Input: part model. Units: mm. Frame: model coordinates. Give positions to 0.01 mm unless a question says otherwise; leave off trailing zeros. Order: outer loops, then holes, each group sorted by start corner. A loop starts at its lowest first (then second) coordinate and runs counter-clockwise, first axis right, second up. Notation, with made-up numbers: (-29, -36) - (0, -36) arc R31 cw to (0, -9) - close; hole circle Ø9 at (7, 18.5). An arc over 180 degrees is marked (long way). Use a Markdown table: item, result.
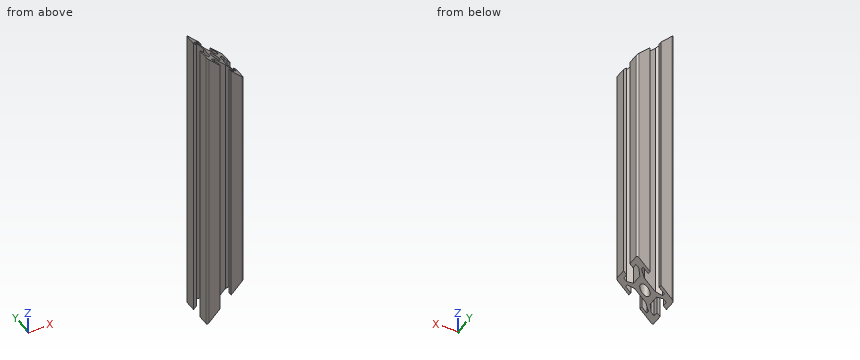
from build123d import *

# Parameters (mm, degrees)
BOSS_EXTRUDE1_DEPTH     = 82.23
CUT_EXTRUDE1_DEPTH      = 166.066930668
CUT_EXTRUDE1_DEPTH_BACK = 166.066930668
SKETCH2_R               = 2.5
FILLET1_R               = 1
SKETCH3_W               = 42.278905999
SKETCH3_H               = 22
CUT_EXTRUDE2_DEPTH      = 128.405385483
SKETCH4_W               = 35
SKETCH4_H               = 22.104489803
CUT_EXTRUDE3_DEPTH      = 128.405385483


with BuildPart() as part:
    # Sketch1 → Boss-Extrude1 (new, symmetric)
    with BuildSketch(Plane.XY):
        Polygon((-10, 10), (-3, 10), (-3, 8.272610059), (-5.783778863, 8.272610059), (-5.783778863, 6.747994248), (-3, 4.550753814), (3, 4.550753814), (5.783778863, 6.747994248), (5.783778863, 8.272610059), (3, 8.272610059), (3, 10), (10, 10), (10, 3), (8.272610059, 3), (8.272610059, 5.783778863), (6.747994248, 5.783778863), (4.55, 3.000595152), (4.55, -2.999404848), (6.747994248, -5.783778863), (8.272610059, -5.783778863), (8.272610059, -3), (10, -3), (10, -10), (3, -10), (3, -8.272610059), (5.783778863, -8.272610059), (5.783778863, -6.747994248), (2.999404848, -4.55), (-3.000595152, -4.55), (-5.783778863, -6.747994248), (-5.783778863, -8.272610059), (-3, -8.272610059), (-3, -10), (-10, -10), (-10, -3), (-8.272610059, -3), (-8.272610059, -5.783778863), (-6.747994248, -5.783778863), (-4.55, -3.000595152), (-4.55, 2.999404848), (-6.747994248, 5.783778863), (-8.272610059, 5.783778863), (-8.272610059, 3), (-10, 3), align=None)
    extrude(amount=BOSS_EXTRUDE1_DEPTH, both=True)

    # Sketch2 → Cut-Extrude1 (cut, two sides: drawn at the far end of the back side and taken through both)
    with BuildSketch(Plane.XY.offset(82.23).offset(-CUT_EXTRUDE1_DEPTH_BACK)):
        Circle(SKETCH2_R)
    extrude(amount=CUT_EXTRUDE1_DEPTH + CUT_EXTRUDE1_DEPTH_BACK, mode=Mode.SUBTRACT)

    # Fillet1
    fillet1_edges = [part.edges().sort_by_distance(p)[0] for p in [
        (-10, 10, 0),
        (10, 10, 0),
        (10, -10, 0),
        (-10, -10, 0),
    ]]
    fillet(fillet1_edges, radius=FILLET1_R)

    # Sketch3 → Cut-Extrude2 (cut, through all)
    with BuildSketch(Plane(origin=(36.115, 0, -36.115), x_dir=(0.7071067811865477, 0, 0.7071067811865475), z_dir=(-0.7071067811865475, 0, 0.7071067811865477))):
        with Locations((-49.240441639, 0.067646977)):
            Rectangle(SKETCH3_W, SKETCH3_H)
    extrude(amount=-CUT_EXTRUDE2_DEPTH, mode=Mode.SUBTRACT)

    # Sketch4 → Cut-Extrude3 (cut, through all)
    with BuildSketch(Plane(origin=(36.115, 0, 36.115), x_dir=(-0.7071067811865477, 0, 0.7071067811865475), z_dir=(-0.7071067811865475, 0, -0.7071067811865477))):
        with Locations((52.605568003, 0.016996688)):
            Rectangle(SKETCH4_W, SKETCH4_H)
    extrude(amount=-CUT_EXTRUDE3_DEPTH, mode=Mode.SUBTRACT)


solid = part.part
1. Section query A-A (y = 0). Return loops of the section in (x, z), then the cut area to 3 significant figures.
Response:
| item | result |
|---|---|
| outline | (-4.55, -76.78) - (-2.5, -74.73) - (-2.5, 74.73) - (-4.55, 76.78) - close; (2.5, -69.73) - (4.55, -67.68) - (4.55, 67.68) - (2.5, 69.73) - close |
| area | 592 mm^2 |
2. Material intervals for line 1 along Y through (x, z) = (5.75, -24.5); line 2 along X through (y, z) = (0, 11.5), sorted ascending.
Response:
| item | result |
|---|---|
| line 1 | y = -10 to -8.27, -6.72 to -4.52, 4.52 to 6.72, 8.27 to 10 |
| line 2 | x = -4.55 to -2.5, 2.5 to 4.55 |
3. Pin query (flat end, axial travel): pin 1 (6.5 mm diameter, centred on x = 0, y = 0, fed in from +Z); pin 2 (8 mm diameter, centred on x = -5.5, y = -2, fed in from -Z); pin 3 (8 mm diameter, centred on x = 7.5, y = -2, fed in from -Z); pin 4 (3 mm diameter, centred on x = -0.5, y = 6.5, fed in from +Z). Return the tip coordinate at first contact, or that it passes through.
Response:
| item | result |
|---|---|
| pin 1 | stops at z = 75.48 |
| pin 2 | stops at z = -81.6 |
| pin 3 | stops at z = -68.73 |
| pin 4 | passes through |
4. Section query B-B (x = 0). Return loops of the section in (y, z), then the cut area to 3 significant figures.
Response:
| item | result |
|---|---|
| outline | (-4.55, -72.23) - (-2.5, -72.23) - (-2.5, 72.23) - (-4.55, 72.23) - close; (2.5, -72.23) - (4.55, -72.23) - (4.55, 72.23) - (2.5, 72.23) - close |
| area | 592 mm^2 |
